Check sheet for the modelled part. Datum: model origin and axes. Units: mm. Round coordinates to 2 decimals unless told otherwise and drop trailing zeros. Order: outer loops, then holes, each group sorted by start corner. A loop starts at its lowest first (then second) coordinate and runs counter-clockwise, first axis right, second up. Notation, with made-up numbers: M 23.25,23.25 L 51.25,23.25 A23 cw 51.25,47.25 Z; hole C 6.25,21 d9. An arc over 180 degrees is marked long. One line per item, written item: value. Start each with the question number.
(1) Depth check by flat-ended pin: pin 1 Ø2 at (x, z) = (-38.5, 0.5) entering from +Y; pin 2 Ø1.3 at (x, z) = (-12, 3) entering from +Y. Enter the tip coordinate at first touch or a pass-through.
(2) Cross-section at B-B, the plane x = 11. Enter the section's corners in (y, z).
(3) Cross-section at C-C, the plane y = -52.5. Enter the section's corners in (x, z).
(4) Cross-section at A-A, the plane y = -32.5. Enter the section's corners in (x, z).
(5) Cross-section at D-D, the plane x = -32. Enter the section's corners in (y, z).
(6) Thickness scan on L1, parallel to X at y = -20, z = 3.45; L2, parallel to X at y = 6, z = 2.4; L3, parallel to Y at x = -16.5, z = 3.9. Record the ranges inside material, lowest first.
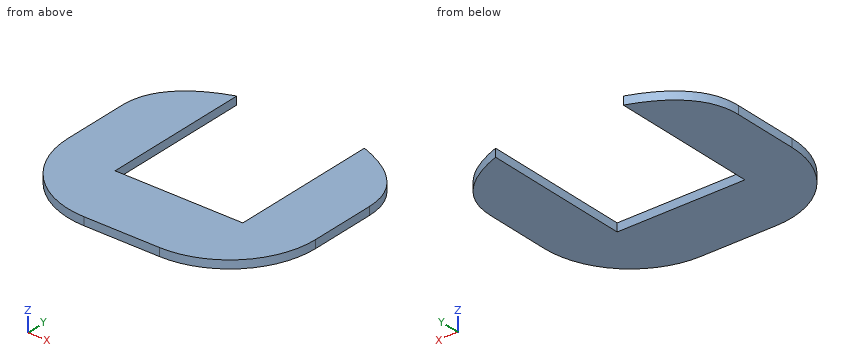
from build123d import *

# Parameters (mm, degrees)
BOSS_EXTRUDE1_DEPTH = 4.3
CUT_EXTRUDE1_DEPTH  = 10


with BuildPart() as part:
    # Sketch1 → Boss-Extrude1 (new body)
    with BuildSketch(Plane.XY):
        with BuildLine():
            Line((-20, -92.2), (-14.429475301, -92.2))
            Line((-14.429475301, -92.2), (20, -92.2))
            ThreePointArc((20, -92.2), (52.3147799, -78.8147799), (65.7, -46.5))
            Line((65.7, -46.5), (65.7, -11.5))
            add(Edge.make_bspline(
                [(65.7, -11.5), (65.7, -10.975589958), (65.677234408, -9.915490978), (65.544187041, -7.888412939), (65.220242618, -5.460671952), (64.598062769, -2.723715825), (63.478515533, 0.7162036), (61.569949009, 4.65452752), (58.553422876, 8.885275051), (54.896250473, 12.662614765), (49.30515895, 17.117750268), (41.279444306, 21.616942397), (32.802615045, 24.780729734), (26.33891585, 26.60624502), (21.797211531, 27.651780938), (17.71021827, 28.4039364), (14.808687361, 28.812738163), (12.872312778, 29.025349646), (11.633648581, 29.131856353), (10.811523275, 29.180203188), (10.282988146, 29.197593371), (10.101212389, 29.2), (10, 29.2)],
                knots=[0, 0, 0, 0, 0.015625, 0.03125, 0.0625, 0.09375, 0.125, 0.1875, 0.25, 0.3125, 0.375, 0.5, 0.625, 0.6875, 0.75, 0.8125, 0.875, 0.90625, 0.9375, 0.96875, 0.984375, 1, 1, 1, 1], degree=3))
            Line((10, 29.2), (-10, 29.2))
            add(Edge.make_bspline(
                [(-10, 29.2), (-10.101212389, 29.2), (-10.282988146, 29.197593371), (-10.811523275, 29.180203188), (-11.633648581, 29.131856353), (-12.872312778, 29.025349646), (-14.808687361, 28.812738163), (-17.71021827, 28.4039364), (-21.797211531, 27.651780938), (-26.33891585, 26.60624502), (-32.802615045, 24.780729734), (-41.279444306, 21.616942397), (-49.30515895, 17.117750268), (-54.896250473, 12.662614765), (-58.553422876, 8.885275051), (-61.569949009, 4.65452752), (-63.478515533, 0.7162036), (-64.598062769, -2.723715825), (-65.220242618, -5.460671952), (-65.544187041, -7.888412939), (-65.677234408, -9.915490978), (-65.7, -10.975589958), (-65.7, -11.5)],
                knots=[0, 0, 0, 0, 0.015625, 0.03125, 0.0625, 0.09375, 0.125, 0.1875, 0.25, 0.3125, 0.375, 0.5, 0.625, 0.6875, 0.75, 0.8125, 0.875, 0.90625, 0.9375, 0.96875, 0.984375, 1, 1, 1, 1], degree=3))
            Line((-65.7, -11.5), (-65.7, -46.5))
            ThreePointArc((-65.7, -46.5), (-52.3147799, -78.8147799), (-20, -92.2))
        make_face()
    extrude(amount=BOSS_EXTRUDE1_DEPTH)

    # Sketch2 → Cut-Extrude1 (cut)
    with BuildSketch(Plane.XY.offset(4.3)):
        Polygon((-33.87, 24.299748656), (-33.87, -54.880251344), (33.87, -54.880251344), (33.87, 24.299748656), (33.87, 35.468874446), (-33.87, 35.468874446), align=None)
    extrude(amount=-CUT_EXTRUDE1_DEPTH, mode=Mode.SUBTRACT)


solid = part.part
Values found:
1. pin 1: y = 22.94
1. pin 2: y = -54.88
2. outline: M -92.2,0 L -54.88,0 L -54.88,4.3 L -92.2,4.3 Z
3. outline: M -65.3,0 L -33.87,0 L -33.87,4.3 L -65.3,4.3 Z; M 33.87,0 L 65.3,0 L 65.3,4.3 L 33.87,4.3 Z
4. outline: M -65.7,0 L -33.87,0 L -33.87,4.3 L -65.7,4.3 Z; M 33.87,0 L 65.7,0 L 65.7,4.3 L 33.87,4.3 Z
5. outline: M -90.6,0 L -54.88,0 L -54.88,4.3 L -90.6,4.3 Z
6. L1: -65.7 to -33.87, 33.87 to 65.7
6. L2: -60.55 to -33.87, 33.87 to 60.55
6. L3: -92.2 to -54.88
